from build123d import *

# Parameters (mm, degrees)
CHAMFER_1_SIZE = 1
CHAMFER_2_SIZE = 1


with BuildPart() as part:
    # 草图1 → 旋转1 (revolve)
    with BuildSketch(Plane(origin=(0, 0, 0), x_dir=(0, 0, -1), z_dir=(1, 0, 0))):
        Polygon((0, 0), (0, 30), (148, 30), (148, 35), (2266, 35), (2266, 30), (2461, 30), (2461, 0), align=None)
    revolve(axis=Axis((0, 0, 0), (0, 0, -1)))

    # 倒角1
    chamfer_1_edges = [part.edges().sort_by_distance(p)[0] for p in [
        (0, -30, -2461),
    ]]
    chamfer(chamfer_1_edges, length=CHAMFER_1_SIZE)

    # 倒角2
    chamfer_2_edges = [part.edges().sort_by_distance(p)[0] for p in [
        (0, -30, 0),
    ]]
    chamfer(chamfer_2_edges, length=CHAMFER_2_SIZE)


solid = part.part
The model under review builds one solid part; all positions refer to its coordinate system, in mm. A direction names the side the tool comes from. Coordinates: 2 decimals unless noted, no trailing zeros. Loops run counter-clockwise (first coordinate to the right, second up) from the corner with the lowest first, then second, coordinate; pieces in that order, holes last.
(1) Wall thickness on L1, parallel to Y at x = 19, z = -1244.5; L2, parallel to X at y = -4.5, z = -379.5; L3, parallel to X at y = -18, z = -945.5: over which ranges is each line inside the solid? List them lowest first.
Determined:
L1: y = -29.39 to 29.39
L2: x = -34.71 to 34.71
L3: x = -30.02 to 30.02
(2) Consider section A-A, the plane y = 0. Give the boundary of the cut face in (x, z).
Determined:
outline: (-35, -2266) - (-30, -2266) - (-30, -2460) - (-29, -2461) - (29, -2461) - (30, -2460) - (30, -2266) - (35, -2266) - (35, -148) - (30, -148) - (30, -1) - (29, 0) - (-29, 0) - (-30, -1) - (-30, -148) - (-35, -148) - close
(3) Tool access review of faces 1 (the flat face through (0, 0, -2461)), 2 (the flat face through (16, 26, -2266)), 3 (the flat face through (16, -26, -148)): name each direction out of +Z, -Z, +X, -X, +Y, -Y from which nothing blocks a thin tool from reaching the whole face with its end or side.
Determined:
face 1: -Z, +X, -X, +Y, -Y
face 2: -Z
face 3: +Z
(4) Consider section C-C, the plane z = -659.5. Give the boundary of the cut face in (x, y).
Determined:
outline: circle Ø70 at (0, 0)
(5) Insertion check: P1, Ø4, axis at x = 9.5, y = -1, coming from the +Z side; P2, Ø5, axis at x = -17, y = 27.5, coming from the -Z side; P3, Ø8, axis at y = -26.5, z = -2152, coming from the +X side; P4, Ø4, axis at x = -26, z = -1276, coming from the +Y side. Each pin has a flat end and moves straight along its axis. Give the tip position at first contact, or say it passes through.
Determined:
P1: stops at z = 0
P2: stops at z = -2460.17
P3: stops at x = 26.81
P4: stops at y = 25.48
